The listing builds one solid part. Answer for the finished solid, in the listing's coordinates (mm). A direction names the side the tool comes from. Give positions to 0.01 mm unless a question says otherwise; leave off trailing zeros. Order: outer loops, then holes, each group sorted by start corner. A loop starts at its lowest first (then second) coordinate and runs counter-clockwise, first axis right, second up. Notation, with made-up numbers: (82, 6) - (88, 6) arc R16 ccw to (88, 27) - close; hole circle Ø3 at (40, -19.5). An arc over 180 degrees is marked (long way). Use CSV: the item, a comma, the result in double quotes.
```python
from build123d import *

# Parameters (mm, degrees)
F0_R      = 6.3637373436
F1_DEPTH  = 6.096
F2_R      = 3.4022099148
F3_DEPTH  = 12.7
F5_R      = 10.1544070979
F6_DEPTH  = 2.54
F8_R      = 5.1242922549
F9_DEPTH  = 8.89
F12_DEPTH = 7.874
F13_D     = 10.16
F13_DEPTH = 1.27
F13_TIP   = 3.0523719447
F14_R     = 1.3490625387
F15_SIZE  = 1.27


with BuildPart() as f1:
    # F0 (on Top) → F1 (new body)
    with BuildSketch(Plane.XY):
        Circle(F0_R)
    extrude(amount=F1_DEPTH)

    # F2 (on Top) → F3 (join)
    with BuildSketch(Plane.XY):
        Circle(F2_R)
    extrude(amount=F3_DEPTH)

    # F5 (on offset) → F6 (join)
    with BuildSketch(Plane.XY.offset(12.7)):
        Circle(F5_R)
    extrude(amount=F6_DEPTH)

    # F8 (on offset) → F9 (join)
    with BuildSketch(Plane.XY.offset(15.24)):
        Circle(F8_R)
    extrude(amount=F9_DEPTH)

    # F11 (on offset) → F12 (cut)
    with BuildSketch(Plane.XY.offset(24.13)):
        with BuildLine():
            Line((1.2634341, 0), (1.2634341, 2.9752182418))
            ThreePointArc((1.2634341, 2.9752182418), (-3.2323659, 0), (1.2634341, -2.9752182418))
            Line((1.2634341, -2.9752182418), (1.2634341, 0))
        make_face()
    extrude(amount=-F12_DEPTH, mode=Mode.SUBTRACT)

    # F13
    with Locations(Plane(origin=(0, 0, 0), x_dir=(1, 0, 0), z_dir=(0, 0, -1))):
        with Locations((0, 0)):
            Hole(F13_D / 2, depth=F13_DEPTH)
            with Locations((0, 0, -(F13_DEPTH + F13_TIP / 2))):  # 118° drill point
                Cone(0, F13_D / 2, F13_TIP, mode=Mode.SUBTRACT)

    # F14
    f14_edges = [f1.edges().sort_by_distance(p)[0] for p in [
        (-6.363737, 0, 6.096),
    ]]
    fillet(f14_edges, radius=F14_R)

    # F15
    f15_edges = [f1.edges().sort_by_distance(p)[0] for p in [
        (-10.154407, 0, 12.7),
    ]]
    chamfer(f15_edges, length=F15_SIZE)


solid = f1.part
```
Item 1: Each of these flat-tipped pins is pushed along its axis until it touches: pin 1 (12 mm diameter, centred on y = 1, z = 4, fed in from +X); pin 2 (2 mm diameter, centred on x = 1, z = 11, fed in from -Y); pin 3 (3 mm diameter, centred on x = -2.5, y = -6.5, fed in from +Z). Where does it stop, or does it pass through?
Taken from the geometry:
pin 1,"x = 6.36"
pin 2,"y = -3.4"
pin 3,"z = 15.24"
Item 2: The part is cut by section A-A (z = 19.25). Give the vertices of the cut face in (x, y).
Taken from the geometry:
outline,"circle Ø10.25 at (0, 0); hole (1.26, -2.98) - (1.26, 2.98) arc R3.23 ccw (long way) to start"
Item 3: Find the intervals of material crossed by line 1 along Y through (x, z) = (0, 21); line 2 along Y through (x, z) = (0, 0.9); line 3 along Z through (x, y) = (1.75, 4), in increasing order.
Taken from the geometry:
line 1,"-5.12 to -3.23, 3.23 to 5.12"
line 2,"-6.36 to -5.08, 5.08 to 6.36"
line 3,"1.7 to 6.1, 12.7 to 24.13"
Item 4: Which of the six approach directions +Z, -Z, +X, -X, +Y, -Y give full straight-line access (tool end or side, diameter ignored) to faces 4 (the face through (-1.38, -6.212, 2.34)), 5 (the face through (1.263, 0, 20)), 6 (the face through (2, 0, 24.13))?
Taken from the geometry:
face 4,"-Z"
face 5,"+Z"
face 6,"+Z, +X, -X, +Y, -Y"
Item 5: The part is cut by section B-B (z = 10.5). Give the vertices of the cut face in (x, y).
Taken from the geometry:
outline,"circle Ø6.8 at (0, 0)"
Item 6: The mould has two halves that part along Y. Classify faces 1 (the face through (0.661, -5.037, 0.644)), 2 (the face through (3.143, -1.303, 9.352)), 3 (the face through (4, 0, 12.7)): +Y half, -Y half, draft (parallel to the pull), parting line (faces both ways), or undercut.
Taken from the geometry:
face 1,"undercut"
face 2,"parting line"
face 3,"draft"
